CAD build for the part. Positions are in the model's coordinates, mm. Face numbers are marked on the shaded views. A direction names the side the tool comes from. Coordinates: 2 decimals unless noted, no trailing zeros. Loops run counter-clockwise (first coordinate to the right, second up) from the corner with the lowest first, then second, coordinate; pieces in that order, holes last. Notation, with made-up numbers: (31.5, 83.5) -> (75.5, 83.5) arc R18 ccw to (75.5, 100.5) -> close; hole circle Ø4 at (11.5, 9.25). An arc over 180 degrees is marked (long way). Answer as CSV lines item,"result". Start each with the question number.
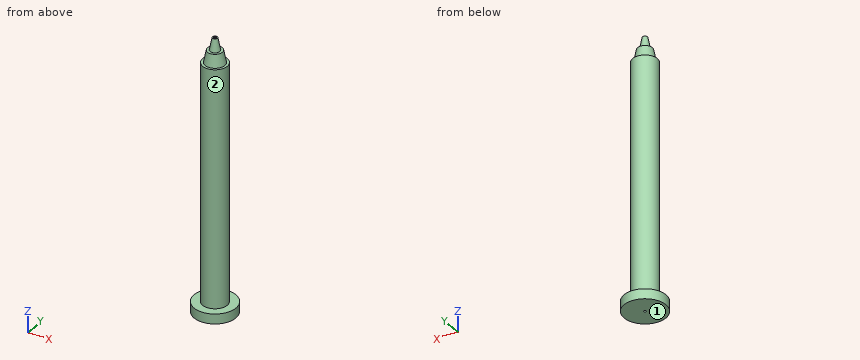
from build123d import *

# Parameters (mm, degrees)
F0_R     = 8.5
F1_DEPTH = 4
F2_R     = 5
F3_DEPTH = 100
F8_R     = 0.5
F9_DEPTH = 125.6


with BuildPart() as f1:
    # F0 (on Top) → F1 (new body)
    with BuildSketch(Plane.XY):
        Circle(F0_R)
    extrude(amount=F1_DEPTH)

    # F2 (on Top) → F3 (join)
    with BuildSketch(Plane.XY):
        Circle(F2_R)
    extrude(amount=F3_DEPTH)

    # F4 (on Right) → F5 (revolve)
    with BuildSketch(Plane.YZ):
        Polygon((3, 105), (0, 105), (0, 100), (4, 100), align=None)
    revolve(axis=Axis((0, 0, 102.5), (0, 0, -1)))

    # F6 (on Right) → F7 (revolve)
    with BuildSketch(Plane.YZ):
        Polygon((1, 110), (0, 110), (0, 105), (2, 105), align=None)
    revolve(axis=Axis((0, 0, 107.5), (0, 0, -1)))

    # F8 (on face) → F9 (cut)
    with BuildSketch(Plane.XY.offset(110)):
        Circle(F8_R)
    extrude(amount=-F9_DEPTH, mode=Mode.SUBTRACT)


solid = f1.part
Item 1: Which spindle directions (+Z, -Z, +X, -X, +Y, -Y) get a long thin tool onto all of the face, cutting with end or side? Do the marked faces 1 and 2. Say none if no direction does.
Item 2: Wall check: probe 1 along Y at (x, z) = (0, 33.5); probe 2 along Z at (x, y) = (-2.5, -6.5); probe 3 along Z at (x, y) = (1, 2.25). Give the ranges that are in metal, low to high.
Item 3: Flat gauge pins, fed straight in: pin 1 Ø1.5 at (x, z) = (4, 86.5) entering from +Y; pin 2 Ø5 at (x, z) = (-1.5, 63) entering from -Y; pin 3 Ø4 at (y, z) = (-6.5, 46.5) entering from -X; pin 4 Ø1.5 at (y, z) = (-6, 65) entering from -X. Where does each tip first touch, or does it go through?
Item 4: Saw through at A-A (z = 8). Write the cut outline in (x, y).
Item 5: Saw through at B-B (y = -7). Write the cut outline in (x, z).
Geometry check:
1,face 1,"-Z, +X, -X, +Y, -Y"
1,face 2,"+Z"
2,probe 1,"-5 to -0.5, 0.5 to 5"
2,probe 2,"0 to 4"
2,probe 3,"0 to 105"
3,pin 1,"y = 3.8"
3,pin 2,"y = -5"
3,pin 3,"x = -2.18"
3,pin 4,"through"
4,outline,"circle Ø10 at (0, 0); hole circle Ø1 at (0, 0)"
5,outline,"(-4.82, 0) -> (4.82, 0) -> (4.82, 4) -> (-4.82, 4) -> close"
